from build123d import *

# Parameters (mm, degrees)
CROQUIS1_W              = 800
CROQUIS1_H              = 800
SALIENTE_EXTRUIR1_DEPTH = 2000
CORTAR_EXTRUIR1_DEPTH   = 20
CHAFL_N1_SIZE           = 30


with BuildPart() as part:
    # Croquis1 → Saliente-Extruir1 (new body)
    with BuildSketch(Plane(origin=(0, 0, 0), x_dir=(1, 0, 0), z_dir=(0, 1, 0))):
        Rectangle(CROQUIS1_W, CROQUIS1_H)
    extrude(amount=SALIENTE_EXTRUIR1_DEPTH)

    # Croquis2 → Cortar-Extruir1 (cut)
    with BuildSketch(Plane.XY.offset(400)):
        with BuildLine():
            Line((-453.105485689, 1895.512731964), (-453.105485689, 82.602501534))
            ThreePointArc((-453.105485689, 82.602501534), (-438.460824748, 47.247162475), (-403.105485689, 32.602501534))
            Line((-403.105485689, 32.602501534), (426.238550511, 32.602501534))
            ThreePointArc((426.238550511, 32.602501534), (461.59388957, 47.247162475), (476.238550511, 82.602501534))
            Line((476.238550511, 82.602501534), (476.238550511, 1895.512731964))
            ThreePointArc((476.238550511, 1895.512731964), (461.59388957, 1930.868071024), (426.238550511, 1945.512731964))
            Line((426.238550511, 1945.512731964), (-403.105485689, 1945.512731964))
            ThreePointArc((-403.105485689, 1945.512731964), (-438.460824748, 1930.868071024), (-453.105485689, 1895.512731964))
        make_face()
        with BuildLine():
            Line((-403.105485689, 1915.512731964), (426.238550511, 1915.512731964))
            ThreePointArc((426.238550511, 1915.512731964), (440.380686134, 1909.654867588), (446.238550511, 1895.512731964))
            Line((446.238550511, 1895.512731964), (446.238550511, 1487.15617354))
            Line((446.238550511, 1487.15617354), (-423.105485689, 1487.15617354))
            Line((-423.105485689, 1487.15617354), (-423.105485689, 1895.512731964))
            ThreePointArc((-423.105485689, 1895.512731964), (-417.247621312, 1909.654867588), (-403.105485689, 1915.512731964))
        make_face(mode=Mode.SUBTRACT)
        with BuildLine():
            Line((-403.105485689, 62.602501534), (426.238550511, 62.602501534))
            ThreePointArc((426.238550511, 62.602501534), (440.380686134, 68.460365911), (446.238550511, 82.602501534))
            Line((446.238550511, 82.602501534), (446.238550511, 1129.448445192))
            Line((446.238550511, 1129.448445192), (-423.105485689, 1129.448445192))
            Line((-423.105485689, 1129.448445192), (-423.105485689, 82.602501534))
            ThreePointArc((-423.105485689, 82.602501534), (-417.247621312, 68.460365911), (-403.105485689, 62.602501534))
        make_face(mode=Mode.SUBTRACT)
    extrude(amount=-CORTAR_EXTRUIR1_DEPTH, mode=Mode.SUBTRACT)

    # Chaflán1
    chafl_n1_edges = [part.edges().sort_by_distance(p)[0] for p in [
        (-400, 2000, 0),
        (400, 2000, 0),
    ]]
    chamfer(chafl_n1_edges, length=CHAFL_N1_SIZE)


solid = part.part
The model under review builds one solid part; all positions refer to its coordinate system, in mm. Round coordinates to 2 decimals unless told otherwise and drop trailing zeros. Order: outer loops, then holes, each group sorted by start corner. A loop starts at its lowest first (then second) coordinate and runs counter-clockwise, first axis right, second up. Notation, with made-up numbers: (54.25, -36) -> (61.25, -36) arc R26 ccw to (61.25, -10) -> close; hole circle Ø10 at (8.5, -29.5). An arc over 180 degrees is marked (long way). Write item = value, one per line. Start each with the question number.
Item 1: Clearance check with a flat-ended pin moving along its axis: pin 1 Ø24 at (x, y) = (65.5, 1929.5) entering from +Z. State where the tip first meets the part, or that it passes through.
Item 2: For line 1 along Z through (x, y) = (-300.5, 1428), list the stretches that pass through material, from the lowest coordinate up.
Item 3: Consider section A-A on y = 1376.5. Write out the cut boundary in (x, z), plus the area to 3 significant figures.
Item 4: Mouldability with a two-part tool opening along Y and no side actions: class faces 1 (the face through (-6, 1311, 380)), 2 (the face through (-5, 2000, -6)), 3 (the face through (-6, 0, -6)), 4 (the face through (-6, 1698, 400)) as released by +Y, released by -Y, zero draft, split by the parting line, or undercut.
Conclusion:
q1.pin_1 = 380
q2.line_1 = -400 to 380
q3.outline = (-400, -400) -> (400, -400) -> (400, 380) -> (-400, 380) -> close
q3.area = 624,000 mm2
q4.face_1 = undercut
q4.face_2 = released by +Y
q4.face_3 = released by -Y
q4.face_4 = zero draft
